Autodesk Inventor part; units mm, degrees
ref_plane "YZ Plane" through (0, 0, 0) normal (1, 0, 0) x (0, 1, 0)
ref_plane "XZ Plane" through (0, 0, 0) normal (0, 1, 0) x (-1, 0, 0)
ref_plane "XY Plane" through (0, 0, 0) normal (0, 0, 1) x (1, 0, 0)
sketch "Sketch1" plane through (0, 0, 0) normal (0, 1, 0) x (-1, 0, 0)
  circle A0 centre (0, 0) radius 6
  dimension "d0" = 12
extrude "Extrusion1" add sketch "Sketch1" along normal mid plane 6
sketch "Sketch2" plane through (0, 3, 0) normal (0, 1, 0) x (1, 0, 0)
  circle A0 centre (0, 0) radius 4
  dimension "d3" = 8
extrude "Extrusion2" add sketch "Sketch2" along normal blind 5
sketch "Sketch3" plane through (0, 8, 0) normal (0, 1, 0) x (1, 0, 0)
  circle A0 centre (0, 0) radius 6
  dimension "d6" = 12
extrude "Extrusion3" add sketch "Sketch3" along normal blind 11
sketch "Sketch4" plane through (0, 19, 0) normal (0, 1, 0) x (1, 0, 0)
  circle A0 centre (0, 0) radius 8
  dimension "d9" = 16
extrude "Extrusion4" add sketch "Sketch4" along normal blind 82
sketch "Sketch5" plane through (0, 101, 0) normal (0, 1, 0) x (1, 0, 0)
  circle A0 centre (0, 0) radius 6
  dimension "d12" = 12
extrude "Extrusion5" add sketch "Sketch5" along normal blind 10
sketch "Sketch6" plane through (0, 111, 0) normal (0, 1, 0) x (1, 0, 0)
  circle A0 centre (0, 0) radius 9
  dimension "d15" = 18
extrude "Extrusion6" add sketch "Sketch6" along normal blind 24
sketch "Sketch7" plane through (0, 0, 0) normal (1, 0, 0) x (0, 1, 0)
  circle A0 centre (123, 0) radius 3
  line L0 (111, -9) -> (111, 9)
  point P0 (0, 0)
  dimension "d18" = 6
  dimension "d19" = 12
extrude "Extrusion7" cut sketch "Sketch7" along normal mid plane 24
properties part number "Pieza09_Tornillo" material "Steel"
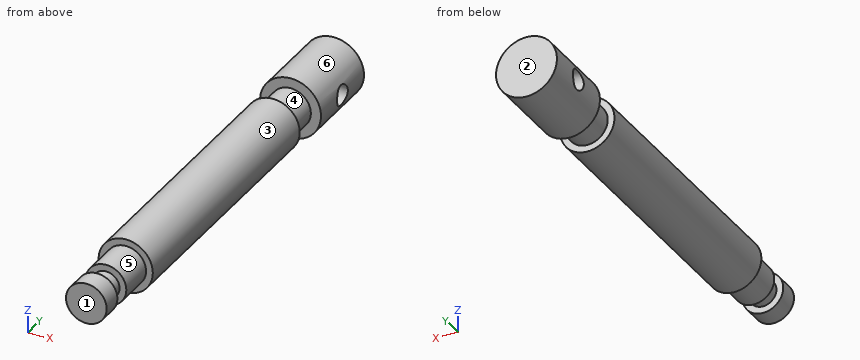
Could you check a few things on this model? Use its own coordinates, in mm. Face numbers are marked on the shaded views. A direction names the side the tool comes from. Coordinates: 2 decimals unless noted, no trailing zeros. Order: outer loops, then holes, each group sorted by start corner. A loop starts at its lowest first (then second) coordinate and runs counter-clockwise, first axis right, second up. Notation, with made-up numbers: (19.25, -3.5) -> (44.25, -3.5) arc R32 cw to (44.25, 23.5) -> close; hole circle Ø4 at (-1.75, 22). An arc over 180 degrees is marked (long way). One line per item, written item: value. Start each with the question number.
1) Imagine slicing it at C-C on y = 42.5. List the corners of the cut face in (x, z) for me.
2) Imagine slicing it at B-B on x = 0. List the corners of the cut face in (y, z) for me.
3) Imagine slicing it at A-A on z = 0. List the corners of the cut face in (x, y) for me, plus the area to 3 significant figures.
4) Imagine slicing it at D-D on y = 123. List the corners of the cut face in (x, z) for me.
5) Which directions (+Z, -Z, +X, -X, +Y, -Y) give clear straight access to the entire face, cutting with the end or side of a thin tool? Please do the marked faces 5 and 6.
6) We'd pull the mould along Y, two halves only. Please class the marked faces 1, 2, 3 and 4: +Y half, -Y half, draft (parallel to the pull), parting line (faces both ways), or undercut.
7) If I drill on L1, parallel to Y at x = 5, z = 0; L2, parallel to Y at x = -4.5, z = 2.5; L3, parallel to Y at x = -5.75, z = 4.25, over which ranges is the centre line in solid material (lowest first)? Write a range as [from, to].
8) I'm going to push flat-ended pins straight in: pin 1 (5.5 mm diameter, centred on x = 4.5, z = 4, fed in from -Y); pin 2 (3 mm diameter, centred on y = 90, z = 1.5, fed in from -X); pin 3 (6 mm diameter, centred on x = 3.5, y = 17.5, fed in from -Z); pin 4 (8 mm diameter, centred on x = -7, y = 37.5, fed in from -Z). Where does each tip first touch, or does it pass through?
Answer list:
1. outline: circle Ø16 at (0, 0)
2. outline: (-3, -6) -> (3, -6) -> (3, -4) -> (8, -4) -> (8, -6) -> (19, -6) -> (19, -8) -> (101, -8) -> (101, -6) -> (111, -6) -> (111, -9) -> (135, -9) -> (135, 9) -> (111, 9) -> (111, 6) -> (101, 6) -> (101, 8) -> (19, 8) -> (19, 6) -> (8, 6) -> (8, 4) -> (3, 4) -> (3, 6) -> (-3, 6) -> close; hole circle Ø6 at (123, 0)
3. outline: (-9, 111) -> (-6, 111) -> (-6, 101) -> (-8, 101) -> (-8, 19) -> (-6, 19) -> (-6, 8) -> (-4, 8) -> (-4, 3) -> (-6, 3) -> (-6, -3) -> (6, -3) -> (6, 3) -> (4, 3) -> (4, 8) -> (6, 8) -> (6, 19) -> (8, 19) -> (8, 101) -> (6, 101) -> (6, 111) -> (9, 111) -> (9, 120) -> (-9, 120) -> close; (-9, 126) -> (9, 126) -> (9, 135) -> (-9, 135) -> close
3. area: 2,000 mm2
4. outline: (-8.49, -3) arc R9 ccw to (8.49, -3) -> close; (-8.49, 3) -> (8.49, 3) arc R9 ccw to start
5. face 5: -Y
5. face 6: +Y, -Y
6. face 1: -Y half
6. face 2: +Y half
6. face 3: draft
6. face 4: undercut
7. L1: y = [-3, 3], [8, 120], [126, 135]
7. L2: y = [-3, 3], [8, 121.34], [124.66, 135]
7. L3: y = [19, 101], [111, 135]
8. pin 1: stops at y = -3
8. pin 2: stops at x = -8
8. pin 3: stops at z = -7.95
8. pin 4: stops at z = -7.42
